Part model, mm, in its own coordinate system. A direction names the side the tool comes from. Round coordinates to 2 decimals unless told otherwise and drop trailing zeros. Loops run counter-clockwise (first coordinate to the right, second up) from the corner with the lowest first, then second, coordinate; pieces in that order, holes last. Notation, with made-up numbers: M 70.25,-34 L 95.25,-34 A18 cw 95.25,-2 Z; hole C 51.25,83.5 d10. An arc over 180 degrees is marked long. Put each result on its own line as item: value. Start each with the question number.
1) Slice it at D-D on z = 67. Give the cut face in (x, y).
2) Which spindle directions (+Z, -Z, +X, -X, +Y, -Y) get a long thin tool onto all of the face, cutting with end or side? Do faces 1 (the flat face through (0, -13, 56)), 2 (the flat face through (-38, -13, 69.705)). Say none if no direction does.
3) Slice it at A-A on z = 52. Give the cut face in (x, y).
4) Slice it at B-B on x = -95.25. Give the cut face in (y, z).
5) Pull direction Z, two halves, no side cores. Call faces 3 (the flat face through (-74, -13, 95.105)), 4 (the flat face through (-50.8, -13, 57)), 5 (the flat face through (-74, 0, 58)): +Z half, -Z half, draft (parallel to the pull), parting line (faces both ways), or undercut.
6) Drop a flat-ended pin along its axis: pin 1 Ø10 at (x, z) = (-122.5, 55.5) entering from +Y. Give the stop position or say it passes through.
7) Slice it at C-C on y = -11.25. Give the cut face in (x, z).
8) Probe line 1 along Z through (x, y) = (-95.25, -19.5); line 2 along X through (y, z) = (-11.75, 60.5); line 3 along X through (y, z) = (-11.5, 55). List the from-to ranges inside material, lowest first.
```python
from build123d import *

# Parameters (mm, degrees)
F0_W     = 146.05
F0_H     = 76.2
F1_DEPTH = 25.4
F3_R     = 12.7
F3_W     = 25.4
F3_H     = 25.4
F4_DEPTH = 25.4


with BuildPart() as f1:
    # F0 (on Front) → F1 (new body)
    with BuildSketch(Plane.XZ):
        with Locations((-73.025, 57.004511)):
            Rectangle(F0_W, F0_H)
    extrude(amount=F1_DEPTH)

    # F3 (on face) → F4 (cut)
    with BuildSketch(Plane.XZ.offset(25.4)):
        with Locations((-95.25, 60.107693)):
            Circle(F3_R)
        with Locations((-38.1, 57.004511)):
            Rectangle(F3_W, F3_H)
    extrude(amount=-F4_DEPTH, mode=Mode.SUBTRACT)


solid = f1.part
```
Recorded:
1. outline: M -146.05,-25.4 L -105.92,-25.4 L -105.92,0 L -146.05,0 Z; M -84.58,-25.4 L -50.8,-25.4 L -50.8,0 L -84.58,0 Z; M -25.4,-25.4 L 0,-25.4 L 0,0 L -25.4,0 Z
2. face 1: +Z, -Z, +X, +Y, -Y
2. face 2: +Y, -Y
3. outline: M -146.05,-25.4 L -105.03,-25.4 L -105.03,0 L -146.05,0 Z; M -85.47,-25.4 L -50.8,-25.4 L -50.8,0 L -85.47,0 Z; M -25.4,-25.4 L 0,-25.4 L 0,0 L -25.4,0 Z
4. outline: M -25.4,18.9 L 0,18.9 L 0,47.41 L -25.4,47.41 Z; M -25.4,72.81 L 0,72.81 L 0,95.1 L -25.4,95.1 Z
5. face 3: +Z half
5. face 4: undercut
5. face 5: draft
6. pin 1: stops at y = 0
7. outline: M -146.05,18.9 L 0,18.9 L 0,95.1 L -146.05,95.1 Z; hole C -95.25,60.11 d25.4; hole M -50.8,44.3 L -25.4,44.3 L -25.4,69.7 L -50.8,69.7 Z
8. line 1: z = 18.9 to 47.41, 72.81 to 95.1
8. line 2: x = -146.05 to -107.94, -82.56 to -50.8, -25.4 to 0
8. line 3: x = -146.05 to -106.88, -83.62 to -50.8, -25.4 to 0
